```python
from build123d import *

# Parameters (mm, degrees)
F2_R     = 0.45
F3_DEPTH = 100
F4_R     = 0.5
F5_DEPTH = 10


with BuildPart() as f1:
    # F0 (on Right) → F1 (revolve)
    with BuildSketch(Plane.YZ):
        Polygon((-1.19, 0), (0, 0), (0, 15), (-1.05, 15), (-1.19, 14.8), align=None)
    revolve(axis=Axis((0, 0, 7.5), (0, 0, 1)))

    # F2 (on Top) → F3 (cut)
    with BuildSketch(Plane.XY):
        Circle(F2_R)
    extrude(amount=F3_DEPTH, mode=Mode.SUBTRACT)

    # F4 (on face) → F5 (cut)
    with BuildSketch(Plane(origin=(0, 0, 0), x_dir=(1, 0, 0), z_dir=(0, 0, -1))):
        Circle(F4_R)
    extrude(amount=-F5_DEPTH, mode=Mode.SUBTRACT)


solid = f1.part
```
The model under review builds one solid part; all positions refer to its coordinate system, in mm. Give positions to 0.01 mm unless a question says otherwise; leave off trailing zeros. Write each loop counter-clockwise with the first axis right and the second up, starting at its lowest first coordinate (ties: lowest second). Pieces come first, ordered by that corner, then holes. Notation, with made-up numbers: M 43.5,52.5 L 62.5,52.5 A17 cw 62.5,56.5 Z; hole C 68,4 d11. An arc over 180 degrees is marked long. Write each question's results on one line, items separated by ' | '. Start each with the question number.
1. Mouldability with a two-part tool opening along X and no side actions: class faces 1 (the cylindrical face through (0.429, 0.135, 12.465)), 2 (the cylindrical face through (-1.16, 0.26, 7.3)), 3 (the flat face through (0, -1, 0)) as released by +X, released by -X, zero draft, split by the parting line, or undercut.
2. Insertion check: pin 1 Ø1 at (x, z) = (-1, 6) entering from +Y. The pin has a flat end and moves straight along its axis. Give the tip position at first contact, or say it passes through.
3. We need section A-A (x = 0). Write out the cut boundary in (y, z).
4. We need section D-D (z = 13.5). Write out the cut boundary in (x, y), and give its area (3 significant figures).
5. For probe 1 along X at (y, z) = (0, 7); probe 2 along X at (y, z) = (0, 13.4); probe 3 along Y at (x, z) = (0.1, 6.5), list the stretches that pass through material, from the lowest coordinate up. Write a range as [from, to].
6. We need section C-C (z = 5.75). Write out the cut boundary in (x, y), and give its area (3 significant figures).
Results found:
1) face 1: undercut | face 2: split by the parting line | face 3: zero draft
2) pin 1: stops at y = 1.08
3) outline: M -1.19,0 L -0.5,0 L -0.5,10 L -0.45,10 L -0.45,15 L -1.05,15 L -1.19,14.8 Z; M 0.45,10 L 0.5,10 L 0.5,0 L 1.19,0 L 1.19,14.8 L 1.05,15 L 0.45,15 Z
4) outline: C 0,0 d2.38; hole C 0,0 d0.9 | area: 3.81 mm^2
5) probe 1: x = [-1.19, -0.5], [0.5, 1.19] | probe 2: x = [-1.19, -0.45], [0.45, 1.19] | probe 3: y = [-1.19, -0.49], [0.49, 1.19]
6) outline: C 0,0 d2.38; hole C 0,0 d1 | area: 3.66 mm^2
